For this review, take the finished solid that the model builds, in its own axes (mm). A direction names the side the tool comes from. Coordinates: 2 decimals unless noted, no trailing zeros. Loops run counter-clockwise (first coordinate to the right, second up) from the corner with the lowest first, then second, coordinate; pieces in that order, holes last.
1. Clearance check with flat-ended pins moving along their axes: P1, Ø1, axis at y = 1.5, z = 2, coming from the -X side; P2, Ø1, axis at x = 3.5, y = 3, coming from the -Z side; P3, Ø2, axis at x = -2, z = 16, coming from the -Y side. State where each tip first meets the part, or that it passes through.
2. Machinability: for faces 1 (the face through (5, 0, 14)), 2 (the face through (4.445, 3.507, 4.243)), 3 (the face through (-4.4, -3.45, 4.34)), which of the approach directions +Z, -Z, +X, -X, +Y, -Y give a long, thin tool a straight path to every point of the face, cutting with its end or side? Answer none if there is none.
3. Take a section at C-C, the plane z = 4. State the section outline as (x, y) points.
4. To check wall thickness, follow probe 1 along X at (y, z) = (-2, 0); probe 2 along Z at (x, y) = (0, 0.25); probe 3 along Z at (x, y) = (1, 0.75). State the ranges of each line that lie inside material, in increasing order.
5. Take a section at D-D, the plane x = -1.5. State the section outline as (y, z) points.
6. Take a section at A-A, the plane y = 0. State the section outline as (x, z) points, then the cut area to 3 significant figures.
```python
from build123d import *

# Parameters (mm, degrees)
SKETCH2_R           = 5
BOSS_EXTRUDE2_DEPTH = 22.5
BOSS_EXTRUDE3_DEPTH = 5
SKETCH4_R           = 2.5
CUT_EXTRUDE1_DEPTH  = 15


with BuildPart() as part:
    # Sketch2 → Boss-Extrude2 (new body)
    with BuildSketch(Plane.XY):
        with Locations(Location((0, 0, 0), (0, 0, 180))):
            Circle(SKETCH2_R)
    extrude(amount=BOSS_EXTRUDE2_DEPTH)

    # Sketch3 → Boss-Extrude3 (add, symmetric)
    with BuildSketch(Plane(origin=(0, 0, 0), x_dir=(1, 0, 0), z_dir=(0, 1, 0))):
        with BuildLine():
            Line((-4.879396794, -2.229791716), (-4.879396794, 2.229791716))
            ThreePointArc((-4.879396794, 2.229791716), (0, 7.10918851), (4.879396794, 2.229791716))
            Line((4.879396794, 2.229791716), (4.879396794, -2.229791716))
            ThreePointArc((4.879396794, -2.229791716), (0, -7.10918851), (-4.879396794, -2.229791716))
        make_face()
    extrude(amount=BOSS_EXTRUDE3_DEPTH, both=True)

    # Sketch4 → Cut-Extrude1 (cut)
    with BuildSketch(Plane.XZ.offset(5)):
        with Locations(Location((0, 0, 0), (0, 0, 270))):
            Circle(SKETCH4_R)
    extrude(amount=-CUT_EXTRUDE1_DEPTH, mode=Mode.SUBTRACT)


solid = part.part
```
Results list:
1. P1: stops at x = -4.9
1. P2: stops at z = -6.08
1. P3: stops at y = -4.9
2. face 1: +Z
2. face 2: +Z, +X, +Y
2. face 3: +Z, -X, -Y
3. outline: (-4.55, -5) - (4.55, -5) - (4.55, -2.08) arc R5 ccw to (4.55, 2.08) - (4.55, 5) - (-4.55, 5) - (-4.55, 2.08) arc R5 ccw to (-4.55, -2.08) - close
4. probe 1: x = -4.88 to -2.5, 2.5 to 4.88
4. probe 2: z = -7.11 to -2.5, 2.5 to 22.5
4. probe 3: z = -7.01 to -2.29, 2.29 to 22.5
5. outline: (-5, -6.87) - (5, -6.87) - (5, -2) - (-5, -2) - close; (-5, 2) - (5, 2) - (5, 6.87) - (4.77, 6.87) - (4.77, 22.5) - (-4.77, 22.5) - (-4.77, 6.87) - (-5, 6.87) - close
6. outline: (-5, 0) - (-4.88, 0) - (-4.88, -2.23) arc R4.88 ccw to (4.88, -2.23) - (4.88, 0) - (5, 0) - (5, 22.5) - (-5, 22.5) - close; hole circle Ø5 at (0, 0)
6. area: 265 mm2
